The listing builds one solid part. Answer for the finished solid, in the listing's coordinates (mm). Face numbers are marked on the shaded views. Round coordinates to 2 decimals unless told otherwise and drop trailing zeros. Write each loop counter-clockwise with the first axis right and the second up, starting at its lowest first coordinate (ties: lowest second). Pieces come first, ordered by that corner, then holes.
Item 1: Each of these flat-tipped pins is pushed along its axis until it touches: pin 1 (12 mm diameter, centred on x = 8, y = 45.5, fed in from -Z); pin 2 (2 mm diameter, centred on x = 33, z = 5, fed in from +Y); pin 3 (10 mm diameter, centred on x = -20.5, z = 14.5, fed in from -Y). Where does it stop, or does it pass through?
Item 2: Find section C-C on z = -18. Give the vertices of the cut face in (x, y), then the cut area to 3 significant figures.
Item 3: Find section A-A on y = 12. Give the vertices of the cut face in (x, z), then the cut area to 3 significant figures.
Item 4: For a pull along X with two mould halves and no side action, classify the marked faces 1, 2 and 3 as +X half, -X half, draft (parallel to the pull), parting line (faces both ways), or undercut.
Item 5: Find the intervals of material crossed by probe 1 along X at (y, z) = (42, 0); probe 2 along X at (y, z) = (49.5, 1.5), in increasing order.
Item 6: Find section B-B on x = -34.5. Give the vertices of the cut face in (y, z), then the cut area to 3 significant figures.
Autodesk Inventor part; units mm, degrees
ref_plane "YZ Plane" through (0, 0, 0) normal (1, 0, 0) x (0, 1, 0)
ref_plane "XZ Plane" through (0, 0, 0) normal (0, 1, 0) x (-1, 0, 0)
ref_plane "XY Plane" through (0, 0, 0) normal (0, 0, 1) x (1, 0, 0)
sketch "Эскиз1" plane through (0, 0, 0) normal (0, 1, 0) x (-1, 0, 0)
  circle A0 centre (0, 0) radius 11.5
  circle A1 centre (0, 0) radius 14
  dimension "d0" = 23
  dimension "d1" = 28
extrude "Выдавливание1" add sketch "Эскиз1" along normal blind 40
sketch "Эскиз6" plane through (0, 40, 0) normal (0, 1, 0) x (1, 0, 0)
  circle A0 centre (0, 0) radius 14
  circle A1 centre (0, 0) radius 11.5
  circle A2 centre (0, 0) radius 12
  circle A3 centre (0, 0) radius 12
extrude "Выдавливание5" add sketch "Эскиз6" along normal blind 14 contours A0 | A2
ref_plane "РабПлоскость1" through (0, 54, 11.8651) normal (1, 0, 0) x (0, 0, -1)
sketch "Эскиз8" plane through (0, 54, 11.8651) normal (1, 0, 0) x (0, 0, -1)
  line L0 (25.8651, 0) -> (-2.1349, 0)
  point P0 (11.8651, -54)
sketch "Эскиз9" plane through (0, 54, 11.8651) normal (1, 0, 0) x (0, 0, -1)
  line L0 (25.8651, 0) -> (-2.1349, 0)
  line L1 (-2.1349, 0) -> (27.9474, -10)
  line L2 (27.9474, -10) -> (27.9474, 0)
  line L3 (25.8651, -54) -> (25.8651, 0)
  line L4 (27.9474, 0) -> (-2.1349, 0)
  line L5 (0.3651, 0) -> (23.3651, 0)
  point P0 (11.8651, -54)
  dimension "d30" = 10
extrude "Выдавливание7" cut sketch "Эскиз9" along normal mid plane 70
sketch "Эскиз10" plane through (0, 49.3461, 0) normal (0, 0.9489425, -0.3154492) x (1, 0, 0)
  line L0 (50, -30) -> (-50, -30)
  line L1 (-50, -30) -> (-50, 30)
  line L2 (-50, 30) -> (50, 30)
  line L3 (50, 30) -> (50, -30)
  line L4 (50, -30) -> (-50, 30) construction
  line L5 (-50, -30) -> (50, 30) construction
  point P0 (0, 15.5662)
  point P1 (0, 0)
  dimension "d33" = 100
  dimension "d34" = 60
extrude "Выдавливание8" add sketch "Эскиз10" along normal blind 6
sketch "Эскиз11" plane through (0, 55.0397, -1.8927) normal (0, 0.9489425, -0.3154492) x (1, 0, 0)
  circle A0 centre (-43, -23) radius 2.25
  line L0 (-50, 30) -> (-50, -30)
  line L1 (-50, -30) -> (50, -30)
  circle A1 centre (-43, 23) radius 2.25
  line L2 (50, 30) -> (-50, 30)
  circle A2 centre (43, -23) radius 2.25
  line L3 (50, -30) -> (50, 30)
  circle A3 centre (43, 23) radius 2.25
  point P0 (0, 15.5662)
  dimension "d37" = 4.5
  dimension "d38" = 7
  dimension "d39" = 7
  dimension "d40" = 4.5
  dimension "d41" = 7
  dimension "d42" = 7
  dimension "d43" = 4.5
  dimension "d44" = 7
  dimension "d45" = 7
  dimension "d46" = 4.5
  dimension "d47" = 7
  dimension "d48" = 7
extrude "Выдавливание9" cut sketch "Эскиз11" against normal blind 6 contours A0 | A1 | A2 | A3
properties part number "подставка для драйвер хаба"
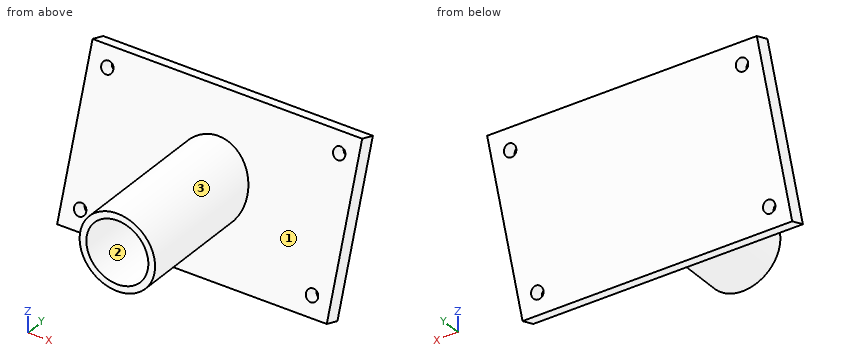
Check values:
1. pin 1: stops at z = -30.36
1. pin 2: stops at y = 57.66
1. pin 3: stops at y = 52.5
2. outline: (-50, 43.36) - (50, 43.36) - (50, 49.69) - (-50, 49.69) - close
2. area: 632 mm2
3. outline: circle Ø28 at (0, 0); hole circle Ø23 at (0, 0)
3. area: 200 mm2
4. face 1: draft
4. face 2: undercut
4. face 3: parting line
5. probe 1: x = -14 to -11.5, 11.5 to 14
5. probe 2: x = -13.92 to -11.4, 11.4 to 13.92
6. outline: (39.88, -28.47) - (45.58, -30.36) - (64.5, 26.58) - (58.81, 28.47) - close
6. area: 360 mm2
